Here's the drawing with two shaded views (mm, measured from the low corner). I have some questions. A direction names the side the tool comes from. Give positions to 0.01 mm unless a question says otherwise; leave off trailing zeros. Write each loop counter-clockwise with the first axis right and the second up, starting at its lowest first coordinate (ties: lowest second). Pieces come first, ordered by that corner, then holes. Notation, with made-up numbers: (33.5, 86) - (79.5, 86) arc R35 ccw to (79.5, 120) - close; hole circle Ø9 at (-35.75, 16). An arc over 180 degrees is marked (long way). Write item = value, one per line.
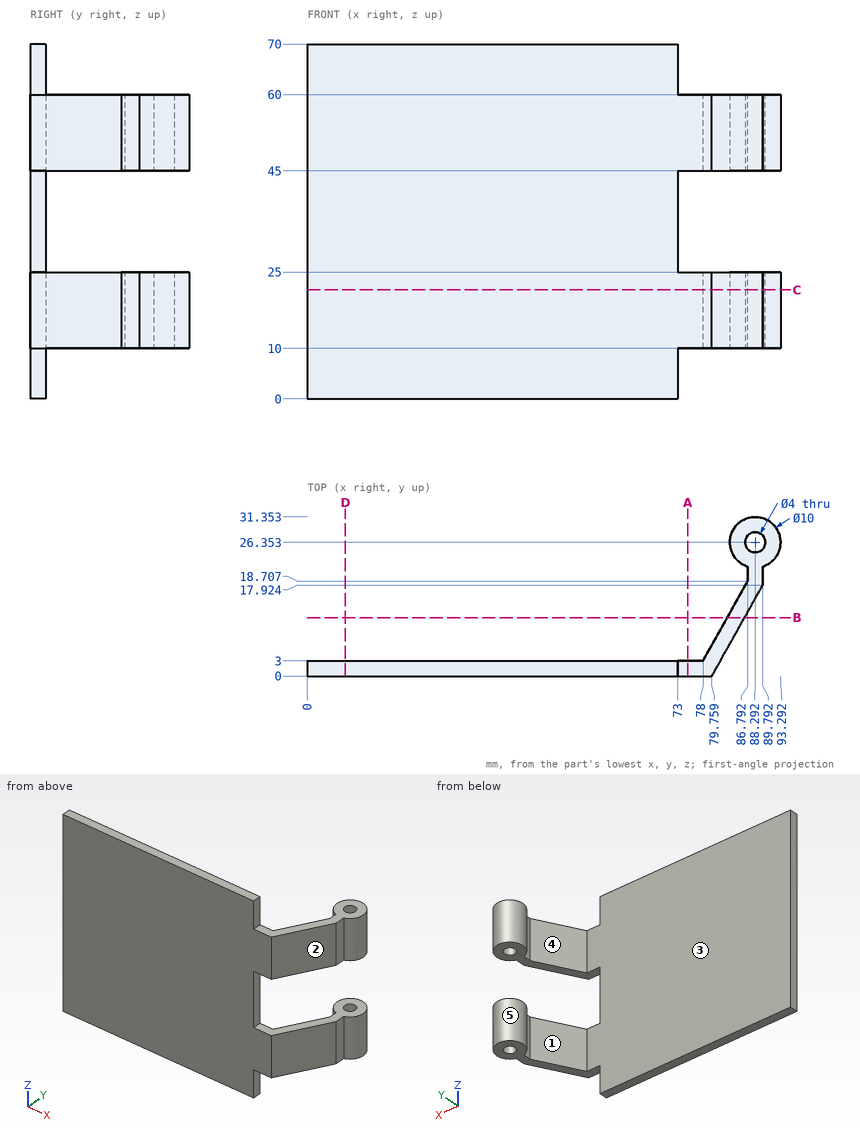
1. If we section it at C-C, the plane z = 21.5: Please give me the cut outline in (x, y) (1 decimal).
Filled sheet:
outline = (0, 0) - (79.8, 0) - (89.8, 17.9) - (89.8, 21.6) arc R5 ccw (long way) to (86.8, 21.6) - (86.8, 18.7) - (78, 3) - (0, 3) - close; hole circle Ø4 at (88.3, 26.4)
2. Thinking about a two-plate mould opening in Y: for the marked faces 1, 2 and 3, which applies, pulls with the +Y half, pulls with the -Y half, needs draft (parallel to the pull), parting line crosses it, or undercut?
Filled sheet:
face_1 = undercut
face_2 = pulls with the -Y half
face_3 = pulls with the +Y half
3. If we section it at B-B, the plane y = 11.5: Please give me the cut outline in (x, z), and give its area (3 significant figures).
Filled sheet:
outline = (82.76, 10) - (86.2, 10) - (86.2, 25) - (82.76, 25) - close; (82.76, 45) - (86.2, 45) - (86.2, 60) - (82.76, 60) - close
area = 103 mm2
4. If we section it at D-D, the plane x = 7.5: Please give me the cut outline in (y, z).
Filled sheet:
outline = (0, 0) - (3, 0) - (3, 70) - (0, 70) - close
5. I need wall thicknesses on line 1 (Y direction, x = 31.5, z = 41); line 2 (X direction, y = 2, z = 29); line 3 (X direction, y = 10.5, z = 20) (1 decimal). Which ranges of each line are inside material? Lowest first, please.
Filled sheet:
line_1 = 0 to 3
line_2 = 0 to 73
line_3 = 82.2 to 85.6
6. If we section it at A-A, the plane x = 75: Please give me the cut outline in (y, z).
Filled sheet:
outline = (0, 10) - (3, 10) - (3, 25) - (0, 25) - close; (0, 45) - (3, 45) - (3, 60) - (0, 60) - close
7. Which directions (+Z, -Z, +X, -X, +Y, -Y) give clear straight access to the entire face, cutting with the end or side of a thin tool? Please do the marked faces 4 and 5.
Filled sheet:
face_4 = +Z, -Z, -X
face_5 = +Z, -Z
8. For pin 1 (21 mm diameter, centred on x = 47.5, z = 42.5, fed in from +Y); pin 2 (1 mm diameter, centred on y = 20.5, z = 47.5, fed in from +X); pin 3 (2.5 mm diameter, centred on y = 20.5, z = 55, fed in from -X), each with a flat end and sliding along its axis, tell me the tip position at first contact or that it passes through.
Filled sheet:
pin_1 = 3
pin_2 = 89.79
pin_3 = 86.34
